Input: part model. Units: mm. Frame: model coordinates. A direction names the side the tool comes from. Round coordinates to 2 decimals unless told otherwise and drop trailing zeros. Loops run counter-clockwise (first coordinate to the right, second up) from the corner with the lowest first, then second, coordinate; pieces in that order, holes last. Notation, with made-up numbers: M 8.5,-15 L 42.5,-15 A23 cw 42.5,13 Z; hole C -28.5,5 d1. An arc over 180 degrees is marked long. Use one line per item in the form item = value. Start each with the question number.
Q1. Section query C-C, the plane x = -57.5. Output: boundary loops of the cut face in (y, z), and give its area (3 significant figures).
Q2. Access query for faces 1 (the cylindrical face through (-50.49, -9.93, 2.85)), 2 (the cylindrical face through (-50.65, 9.93, 3.01)), 3 (the cylindrical face through (-50.65, -9.93, 16.99)), 4 (the cylindrical face through (-50.49, 9.93, 17.15)), 5 (the flat face through (81, -5, 12)). Directions: +Z, -Z, +X, -X, +Y, -Y. A direction counts if a zero-diameter tool reaches every point of the face in a straight line with its end or side. Return the directions, or none.
Q3. Mould query, pull axis X, two halves, no side actions, for faces 6 (the cylindrical face through (90.49, 10.07, 17.15)), 7 (the cylindrical face through (82, 10, 8)), 8 (the flat face through (9, 0, 0)). Classes: pulls with the +X half, pulls with the -X half, needs draft (parallel to the pull), parting line crosses it, or undercut.
Q4. First-contact query: P1, Ø4.5, axis at x = 83.5, z = 10, coming from the +Y side; P2, Ø6, axis at x = -60, z = 15, coming from the +Y side; P3, Ø6, axis at x = -57, z = 14, coming from the -Y side. Flat tips, straight axial feed; report the tip coordinate or a pass-through.
Q5. Section query D-D, the plane z = 1.5. Output: boundary loops of the cut face in (x, y).
Q6. Section query B-B, the plane z = 14. Output: boundary loops of the cut face in (x, y), and give its area (3 significant figures).
Q7. Ray query, line 1 along Z through (x, y) = (83.5, 12.75); line 2 along Y through (x, z) = (83, 7.5); line 3 along Y through (x, z) = (-60, 17.25). Return the intervals inside material, ascending.
Solid Edge part; units mm, degrees
sketch "Sketch1" plane through (0, 0, 0) normal (0, 0, 1) x (1, 0, 0)
  line L0 (-53.5, -15) -> (93.5, -15)
  line L1 (93.5, -15) -> (93.5, -5)
  line L2 (93.5, -5) -> (73.5, -5)
  line L3 (73.5, -5) -> (73.5, 5)
  line L4 (73.5, 5) -> (93.5, 5)
  line L5 (93.5, 5) -> (93.5, 15)
  line L6 (93.5, 15) -> (-53.5, 15)
  line L7 (-53.5, 15) -> (-53.5, 5)
  line L8 (-53.5, 5) -> (-73.5, 5)
  line L9 (-73.5, 5) -> (-73.5, -5)
  line L10 (-53.5, -5) -> (-73.5, -5)
  line L11 (-53.5, -15) -> (-53.5, -5)
extrude "Protrusion1" add sketch "Sketch1" along normal blind 20
sketch "Sketch2" plane through (0, -15, 10) normal (0, -1, 0) x (1, 0, 0)
  circle A0 centre (83.5, 0) radius 2.5
  circle A1 centre (-63.501, 0) radius 2.5
extrude "Cutout1" cut sketch "Sketch2" against normal through all
fillet "Redondeo_1" radius 10 6 edges at (-73.5, 0, 20) (93.5, -10, 20) (93.5, -10, 0) (-73.5, 0, 0) (93.5, 10, 20) (93.5, 10, 0)
fillet "Redondeo_2" radius 10 4 edges at (-53.5, -10, 20) (-53.5, 10, 20) (-53.5, 10, 0) (-53.5, -10, 0)
Results found:
q1.outline = M -5,0 L 5,0 L 5,20 L -5,20 Z
q1.area = 200 mm²
q2.face_1 = -Z, -X, -Y
q2.face_2 = -Z, -X, +Y
q2.face_3 = +Z, -X, -Y
q2.face_4 = +Z, -X, +Y
q2.face_5 = +Z, -Z, +X
q3.face_6 = pulls with the +X half
q3.face_7 = undercut
q3.face_8 = needs draft
q4.P1 = through
q4.P2 = 5
q4.P3 = -5
q5.outline = M -68.77,-5 L -48.77,-5 L -48.77,-15 L 88.77,-15 L 88.77,-5 L 73.5,-5 L 73.5,5 L 88.77,5 L 88.77,15 L -48.77,15 L -48.77,5 L -68.77,5 Z
q6.outline = M -72.67,-5 L -52.67,-5 L -52.67,-15 L 92.67,-15 L 92.67,-5 L 73.5,-5 L 73.5,5 L 92.67,5 L 92.67,15 L -52.67,15 L -52.67,5 L -72.67,5 Z
q6.area = 4,370 mm²
q7.line_1 = 0 to 7.5, 12.5 to 20
q7.line_2 = -15 to -5, 5 to 15
q7.line_3 = -5 to 5
